from build123d import *

# Parameters (mm, degrees)
F0_W     = 12.5
F0_H     = 23.2
F1_DEPTH = 22
F3_DEPTH = 5


with BuildPart() as f1:
    # F0 (on Top) → F1 (new body)
    with BuildSketch(Plane.XY):
        with Locations((-7.3471718132, 13.4849312573)):
            Rectangle(F0_W, F0_H)
    extrude(amount=F1_DEPTH)

    # F2 (on face) → F3 (join)
    with BuildSketch(Plane.XY.offset(22)):
        with BuildLine():
            ThreePointArc((-5.7571718132, 19.2849312573), (-7.3471718132, 20.8749312573), (-8.9371718132, 19.2849312573))
            Line((-8.9371718132, 19.2849312573), (-5.7571718132, 19.2849312573))
        make_face()
        with BuildLine():
            Line((-5.7571718132, 19.2849312573), (-8.9371718132, 19.2849312573))
            ThreePointArc((-8.9371718132, 19.2849312573), (-7.3471718132, 17.6949312573), (-5.7571718132, 19.2849312573))
        make_face()
    extrude(amount=F3_DEPTH)


solid = f1.part
Source: CAD feature listing. Evaluate the final solid. Frame: model axes, mm. A direction names the side the tool comes from. Round coordinates to 2 decimals unless told otherwise and drop trailing zeros. Loops run counter-clockwise (first coordinate to the right, second up) from the corner with the lowest first, then second, coordinate; pieces in that order, holes last. Notation, with made-up numbers: (20, -11) - (25, -11) arc R16 cw to (25, 13) - close; hole circle Ø8 at (25, -36.5). An arc over 180 degrees is marked (long way). Write item = value, one per line. Start each with the question number.
Item 1: Material intervals for line 1 (Z direction, x = -5.25, y = 22.5), sorted ascending.
Item 2: Section query D-D on x = -2.5. Output: boundary loops of the cut face in (y, z), plus the area to 3 significant figures.
Item 3: Reachability of faces 1 (the face through (-6.175, 18.21, 24.465)), 2 (the face through (-7, 14, 0)) from +Z, -Z, +X, -X, +Y, -Y: full face, straight path, thin tool, end or side. Return the list, or none.
Item 4: Section query C-C on y = 18. Output: boundary loops of the cut face in (x, z).
Item 5: Section query B-B on x = -6.75. Output: boundary loops of the cut face in (y, z).
Item 6: Section query A-A on y = 7.5. Output: boundary loops of the cut face in (x, z).
Results list:
q1.line_1 = 0 to 22
q2.outline = (1.88, 0) - (25.08, 0) - (25.08, 22) - (1.88, 22) - close
q2.area = 510 mm²
q3.face_1 = +Z
q3.face_2 = -Z, +X, -X, +Y, -Y
q4.outline = (-13.6, 0) - (-1.1, 0) - (-1.1, 22) - (-6.41, 22) - (-6.41, 27) - (-8.28, 27) - (-8.28, 22) - (-13.6, 22) - close
q5.outline = (1.88, 0) - (25.08, 0) - (25.08, 22) - (20.76, 22) - (20.76, 27) - (17.81, 27) - (17.81, 22) - (1.88, 22) - close
q6.outline = (-13.6, 0) - (-1.1, 0) - (-1.1, 22) - (-13.6, 22) - close
